Autodesk Inventor part; units mm, degrees
ref_plane "YZ Plane" through (0, 0, 0) normal (1, 0, 0) x (0, 1, 0)
ref_plane "XZ Plane" through (0, 0, 0) normal (0, 1, 0) x (-1, 0, 0)
ref_plane "XY Plane" through (0, 0, 0) normal (0, 0, 1) x (1, 0, 0)
sketch "Skizze2" plane through (0, 0, 0) normal (1, 0, 0) x (0, 1, 0)
  line L0 (30.5, 0) -> (0, 0)
  line L1 (0, 0) -> (0, 29)
  line L2 (0, 29) -> (30.5, 29)
  line L3 (30.5, 29) -> (30.5, 0)
  line L4 (0, -5.8) -> (0, 34.8)
  line L5 (-26.8, 0) -> (40.05, 0)
  line L6 (23.5, 2) -> (7, 2)
  line L7 (7, 2) -> (7, 27)
  line L8 (7, 27) -> (23.5, 27)
  line L9 (23.5, 27) -> (23.5, 2)
  point P0 (0, 0)
  dimension "d2" = 30.5
  dimension "d3" = 29
  dimension "d4" = 2
  dimension "d5" = 2
  dimension "d6" = 7
  dimension "d7" = 7
extrude "Extrusion1" add sketch "Skizze2" along normal blind 1.5
sketch "Skizze4" plane through (0, 0, 0) normal (-1, 0, 0) x (0, 0, 1)
  line L0 (27, 7) -> (27, 23.5)
  line L1 (2, 23.5) -> (2, 7)
  line L2 (27, 23.5) -> (2, 23.5)
  line L3 (2, 7) -> (27, 7)
  circle A0 centre (4.25, 26.5) radius 1.25
  circle A1 centre (24.75, 26.5) radius 1.25
  circle A2 centre (4.25, 4) radius 1.25
  circle A3 centre (24.75, 4) radius 1.25
  point P0 (0, 0)
  dimension "d24" = 2.5
  dimension "d25" = 3
  dimension "d28" = 20.5
  dimension "d31" = 22.5
  dimension "d34" = 2.25
extrude "Extrusion2" add sketch "Skizze4" along normal blind 7 contours A0 | A1 | A2 | A3
sketch "Skizze5" plane through (0, 0, 0) normal (-1, 0, 0) x (0, 0, 1)
  line L0 (7.5, 7) -> (21.5, 7)
  line L1 (21.5, 7) -> (21.5, 2)
  line L2 (21.5, 2) -> (7.5, 2)
  line L3 (7.5, 2) -> (7.5, 7)
  line L4 (2, 7) -> (27, 7)
  circle A0 centre (4.25, 4) radius 1.25
  circle A1 centre (24.75, 4) radius 1.25
  line L5 (29, 0) -> (0, 0)
  dimension "d35" = 2
  dimension "d36" = 2
  dimension "d37" = 2
extrude "Extrusion3" cut sketch "Skizze5" against normal through all contours L0 L1 L2 L3
sketch "Skizze6" plane through (0, 0, 0) normal (-1, 0, 0) x (0, 0, 1)
  line L0 (2, 7) -> (7.5, 7)
  line L1 (7.5, 2) -> (7.5, 7)
  line L2 (2, 7) -> (7.5, 7)
  line L3 (7.5, 7) -> (7.5, 6)
  line L4 (7.5, 6) -> (2, 6)
  line L5 (2, 6) -> (2, 7)
  line L6 (27, 7) -> (21.5, 7)
  line L7 (21.5, 7) -> (21.5, 6)
  line L8 (21.5, 6) -> (27, 6)
  line L9 (27, 6) -> (27, 7)
  line L10 (21.5, 7) -> (21.5, 2)
  point P0 (0, 0)
  dimension "d40" = 1
extrude "Extrusion4" cut sketch "Skizze6" against normal through all
sketch "Skizze8" plane through (1.5, 0, 0) normal (1, 0, 0) x (0, 0, -1)
  line L0 (-30, 31.5) -> (1, 31.5)
  line L1 (1, 31.5) -> (1, -1)
  line L2 (1, -1) -> (-30, -1)
  line L3 (-30, -1) -> (-30, 31.5)
  line L4 (-29, 0) -> (0, 0)
  line L5 (0, 0) -> (0, 30.5)
  line L6 (0, 30.5) -> (-29, 30.5)
  line L7 (-29, 30.5) -> (-29, 0)
  line L8 (-29, 30.5) -> (0, 30.5)
  line L9 (0, 30.5) -> (0, 0)
  line L10 (0, 0) -> (-29, 0)
  line L11 (-29, 0) -> (-29, 30.5)
  dimension "d43" = 1
  dimension "d44" = 1
  dimension "d45" = 1
  dimension "d46" = 1
extrude "Extrusion5" add sketch "Skizze8" against normal blind 6.5
sketch "Skizze9" plane through (1.5, -1, -1) normal (0, 0, -1) x (-1, 0, 0)
  line L0 (6.5, 32.5) -> (6.5, 0)
  line L1 (0, 32.5) -> (6.5, 32.5)
  line L2 (0, 0) -> (0, 32.5)
  line L3 (0, 32.5) -> (6.5, 32.5)
  line L4 (6.5, 32.5) -> (6.5, 37.5)
  line L5 (0, 31.7695) -> (0, 32.5)
  line L6 (6.5, 37.5) -> (4.5, 37.5)
  line L7 (3.8504, 36.9054) -> (0.6496, 33.9752)
  arc A0 (0.6496, 33.9752) -> (0, 32.5) centre (2, 32.5) ccw
  line L8 (4.5, 38.3806) -> (4.5, 42.5)
  line L9 (4.5, 42.5) -> (6.5, 42.5)
  line L10 (6.5, 42.5) -> (6.5, 37.5)
  arc A1 (3.8504, 36.9054) -> (4.5, 38.3806) centre (2.5, 38.3806) ccw
  point P0 (1.5, 1)
  point P1 (-0.2652, 33.1379)
  dimension "d58" = 2
  dimension "d60" = 2
  dimension "d61" = 5
  dimension "d62" = 2
  dimension "d63" = 10
extrude "Extrusion6" add sketch "Skizze9" against normal blind 31
sketch "Skizze12" plane through (1.5, -1, -1) normal (0, 0, -1) x (-1, 0, 0)
  circle A0 centre (21.5, 42.5) radius 15
  circle A1 centre (21.5, 42.5) radius 17
  line L0 (4.5, 42.5) -> (4.5, 38.3806)
  line L1 (6.5, 42.5) -> (4.5, 42.5)
  line L2 (4.5, 42.5) -> (38.5, 42.5)
  point P0 (1.5, 1)
  point P1 (36.5, 42.5)
  dimension "d64" = 30
extrude "Extrusion7" add sketch "Skizze12" against normal blind 31 contours A0 L1 A1 L2 picked at (5.4766, 45.0527)
sketch "Skizze13" plane through (1.5, -1, -1) normal (0, 0, -1) x (-1, 0, 0)
  line L0 (0, 0) -> (6.5, 0)
  line L1 (0, 0) -> (35.9872, 51.395)
  arc A0 (38.5, 42.5) -> (4.5, 42.5) centre (21.5, 42.5) ccw
  line L2 (0, 0) -> (0, 32.5)
  arc A1 (38.5, 42.5) -> (35.9872, 51.395) centre (21.5, 42.5) ccw
  arc A2 (36.5, 42.5) -> (6.5, 42.5) centre (21.5, 42.5) ccw
  line L3 (38.5, 42.5) -> (36.5, 42.5)
  arc A3 (36.5, 42.5) -> (34.7206, 49.5862) centre (21.5, 42.5) ccw
  point P0 (1.5, 1)
  dimension "d67" = 35
extrude "Extrusion8" cut sketch "Skizze13" against normal through all
sketch "Skizze14" plane through (1.5, -1, -1) normal (0, 0, -1) x (-1, 0, 0)
  arc A0 (34.7206, 49.5862) -> (6.5, 42.5) centre (21.5, 42.5) ccw
  circle A1 centre (21.5, 42.5) radius 15
  line L0 (34.7206, 49.5862) -> (59.2848, 32.3862)
  line L1 (59.2848, 32.3862) -> (60.5513, 34.195)
  arc A2 (35.9872, 51.395) -> (4.5, 42.5) centre (21.5, 42.5) ccw
  line L2 (60.5513, 34.195) -> (35.9872, 51.395)
  line L3 (34.7206, 49.5862) -> (35.9872, 51.395)
  line L4 (60.5513, 34.195) -> (65.5248, 41.2979)
  line L5 (65.5248, 41.2979) -> (63.8865, 42.445)
  line L6 (63.8865, 42.445) -> (58.913, 35.3422)
  point P0 (1.5, 1)
  dimension "d70" = 90
  dimension "d72" = 2
  dimension "d73" = 17.2
  dimension "d74" = 90
  dimension "d76" = 8.25
extrude "Extrusion9" add sketch "Skizze14" against normal blind 31 contours L3 L2 L1 L0 | L2 L6 L5 L4
sketch "Skizze15" plane through (-62.3865, 41.445, 30) normal (0.819152, 0.5735764, 0) x (0, 0, -1)
  circle A0 centre (26, -4.671) radius 2
  circle A1 centre (5, -4.671) radius 2
  line L0 (31, 0) -> (31, -8.671)
  line L1 (0, -8.671) -> (0, 0)
  line L2 (31, -8.671) -> (0, -8.671)
  point P0 (30, -69.7332)
  point P1 (31, -4.3355)
  dimension "d79" = 4
  dimension "d80" = 4
  dimension "d82" = 5
  dimension "d83" = 4
  dimension "d84" = 4
  dimension "d85" = 5
extrude "Extrusion10" cut sketch "Skizze15" against normal through all
properties part number "Bildschirmhalter"
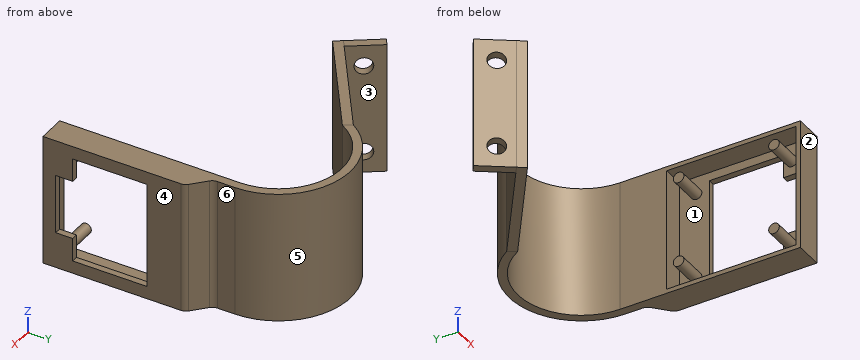
Geometry check sheet. Reference: the model listing, model coordinates, mm. Face numbers are marked on the shaded views. A direction names the side the tool comes from. Round coordinates to 2 decimals unless told otherwise and drop trailing zeros. Loops run counter-clockwise (first coordinate to the right, second up) from the corner with the lowest first, then second, coordinate; pieces in that order, holes last. Notation, with made-up numbers: (29.5, 68.5) -> (74.5, 68.5) arc R29 ccw to (74.5, 89.5) -> close; hole circle Ø1 at (10, 39.25). An arc over 180 degrees is marked (long way). Answer as a JSON object with one key per item and string values. Group by question number.
Item 1: Cross-section at B-B, the plane z = 15. Record the cut outline in (x, y) (1 decimal), plus the area to 3 significant figures.
Item 2: Cross-section at A-A, the plane y = 4. Record the cut outline in (x, z).
Item 3: Cross-section at C-C, the plane y = 26.5. Record the cut outline in (x, z), plus the area to 3 significant figures.
Item 4: Set-up check for the marked faces 5 and 6: record each of +Z, -Z, +X, -X, +Y, -Y from which the full face is reachable in a straight line by a thin tool's end or side.
Item 5: Depth check by flat-ended pin: pin 1 Ø3 at (y, z) = (4, 4) entering from -X; pin 2 Ø1.2 at (x, z) = (1, 16.5) entering from +Y; pin 3 Ø5 at (x, z) = (-50, 12.5) entering from +Y. Enter the tip coordinate at first touch or a pass-through.
Item 6: Thickness scan on line 1 along X through (y, z) = (35, 28.5); line 2 along X through (y, z) = (38.5, 19); line 3 along Z through (x, y) = (-3, 11). Record the ranges inside material, lowest first.
Item 7: Release check for a two-part mould opening along X. For the marked faces 1, 2, 3 and 4 record: pulls with the +X half, pulls with the -X half, needs draft (parallel to the pull), parting line crosses it, or undercut.
Item 8: Cross-section at D-D, the plane y = 43. Record the cut outline in (x, z).
Determined:
{
 "1": {"outline": "(-64, 40.3) -> (-59.1, 33.2) -> (-57.8, 31.4) -> (-33.2, 48.6) arc R15 cw to (-5, 41.5) -> (-5, 30.5) -> (0, 30.5) -> (0, 23.5) -> (1.5, 23.5) -> (1.5, 31.5) arc R2 ccw to (0.9, 33) -> (-2.4, 35.9) arc R2 cw to (-3, 37.4) -> (-3, 41.5) arc R17 ccw to (-34.5, 50.4) -> (-57.4, 34.3) -> (-62.4, 41.4) -> close; (-5, -1) -> (1.5, -1) -> (1.5, 2) -> (0, 2) -> (0, 0) -> (-5, 0) -> close", "area": "227 mm²"},
 "2": {"outline": "(-7, 3) -> (0, 3) -> (0, 0) -> (-5, 0) -> (-5, -1) -> (1.5, -1) -> (1.5, 7.5) -> (0, 7.5) -> (0, 5.5) -> (-7, 5.5) -> close; (-7, 23.5) -> (0, 23.5) -> (0, 21.5) -> (1.5, 21.5) -> (1.5, 30) -> (-5, 30) -> (-5, 29) -> (0, 29) -> (0, 26) -> (-7, 26) -> close"},
 "3": {"outline": "(-7, 3) -> (0, 3) -> (0, 0) -> (-5, 0) -> (-5, -1) -> (1.5, -1) -> (1.5, 30) -> (-5, 30) -> (-5, 29) -> (0, 29) -> (0, 26) -> (-7, 26) -> (-7, 23.5) -> (0, 23.5) -> (0, 5.5) -> (-7, 5.5) -> close", "area": "91.5 mm²"},
 "4": {"face 5": "+Z, -Z, +Y", "face 6": "+Z, -Z, +X, +Y"},
 "5": {"pin 1": "stops at x = -7", "pin 2": "stops at y = 33.39", "pin 3": "stops at y = 41.28"},
 "6": {"line 1": "x = -60.32 to -57.87, -56.47 to -52.62, -5 to -1.36", "line 2": "x = -62.77 to -60.32, -51.47 to -47.63, -5 to -3", "line 3": "z = -1 to 0, 29 to 30"},
 "7": {"face 1": "pulls with the -X half", "face 2": "needs draft", "face 3": "undercut", "face 4": "pulls with the +X half"},
 "8": {"outline": "(-45.05, -1) -> (-41.2, -1) -> (-41.2, 30) -> (-45.05, 30) -> close; (-5.08, -1) -> (-3.07, -1) -> (-3.07, 30) -> (-5.08, 30) -> close"}
}
